```python
from build123d import *

# Parameters (mm, degrees)
FILLET1_R = 2


with BuildPart() as part:
    # Sketch1 → Revolve1 (revolve)
    with BuildSketch(Plane(origin=(0, 0, 0), x_dir=(1, 0, 0), z_dir=(0, 1, 0))):
        with BuildLine():
            Line((-83.333328339, 39.999998202), (-33.392539812, 22.021314332))
            ThreePointArc((-33.392539812, 22.021314332), (11.49561672, 38.312540979), (40, 0))
            Line((40, 0), (-133.33332, 0))
            Line((-133.33332, 0), (-133.33332, 9.999999))
            Line((-133.33332, 9.999999), (-97.73332356, 9.999999))
            Line((-97.73332356, 9.999999), (-97.73332356, 39.999998202))
            Line((-97.73332356, 39.999998202), (-83.333328339, 39.999998202))
        make_face()
    revolve(axis=Axis((25.002810952, 0, 0), (-1, 0, 0)))

    # Fillet1
    fillet1_edges = [part.edges().sort_by_distance(p)[0] for p in [
        (-33.392539812, 0, 22.021314332),
    ]]
    fillet(fillet1_edges, radius=FILLET1_R)


solid = part.part
```
Build history of the part. All positions in model axes, mm. A direction names the side the tool comes from. Round coordinates to 2 decimals unless told otherwise and drop trailing zeros. Order: outer loops, then holes, each group sorted by start corner. A loop starts at its lowest first (then second) coordinate and runs counter-clockwise, first axis right, second up. Notation, with made-up numbers: (-4.75, 48) -> (50.25, 48) arc R13 ccw to (50.25, 62) -> close; hole circle Ø5 at (-28, -4.5). An arc over 180 degrees is marked (long way). Answer in a Markdown table with one row per item.
1) Wall check: L1, parallel to X at y = 15.5, z = -24.5; L2, parallel to Y at x = -92, z = 12; L3, parallel to Y at x = -53, z = -5.5. Give the ranges that are in metal, low to high.
Values:
| item | result |
|---|---|
| L1 | -97.73 to -52.75, -27.56 to 27.56 |
| L2 | -38.16 to 38.16 |
| L3 | -28.56 to 28.56 |
2) Pin check, flat tips, straight feed: P1, Ø1, axis at y = -9, z = -22.5, coming from the +X side; P2, Ø4, axis at x = 3.5, y = 5, coming from the +Z side; P3, Ø10, axis at y = 19, z = 23, coming from the +X side. Stop position of each tip, or through.
Values:
| item | result |
|---|---|
| P1 | x = 32.2 |
| P2 | z = 39.79 |
| P3 | x = 31.36 |
3) Band-saw the part on A-A on x = -95.5. Give the cut face in (y, z).
Values:
| item | result |
|---|---|
| outline | circle Ø80 at (0, 0) |
4) Which spindle directions (+Z, -Z, +X, -X, +Y, -Y) get a long thin tool onto all of the face, cutting with end or side? Do faces 1 (the flat face through (-133.333, 0, 0)), 2 (the cylindrical face through (-115.28, -6.76, 7.37)). Say none if no direction does.
Values:
| item | result |
|---|---|
| face 1 | +Z, -Z, -X, +Y, -Y |
| face 2 | -X |
5) Mould opens along X. For faces 3 (the conical face through (-47.97, -8.19, -26.01)), 4 (the cylindrical face through (-90.43, 39.05, 8.67)), 5 (the flat face through (-97.733, 8, 8)) say: released by +X, released by -X, zero draft, split by the parting line, or undercut.
Values:
| item | result |
|---|---|
| face 3 | undercut |
| face 4 | zero draft |
| face 5 | released by -X |
6) Band-saw the part on B-B on x = -64.5. Give the cut face in (y, z), and give its area (3 significant figures).
Values:
| item | result |
|---|---|
| outline | circle Ø66.44 at (0, 0) |
| area | 3,470 mm2 |
